Geometry: final body of the model. Coordinates: model frame, mm. A direction names the side the tool comes from. Round coordinates to 2 decimals unless told otherwise and drop trailing zeros. Loops run counter-clockwise (first coordinate to the right, second up) from the corner with the lowest first, then second, coordinate; pieces in that order, holes last. Notation, with made-up numbers: (15, -2) - (26, -2) arc R21 cw to (26, 9) - close; hole circle Ø10 at (16.5, 36). An arc over 180 degrees is marked (long way). Answer in a Markdown table with one row per item. Add a question column.
Autodesk Inventor part; units mm, degrees
ref_plane "YZ Plane" through (0, 0, 0) normal (1, 0, 0) x (0, 1, 0)
ref_plane "XZ Plane" through (0, 0, 0) normal (0, 1, 0) x (-1, 0, 0)
ref_plane "XY Plane" through (0, 0, 0) normal (0, 0, 1) x (1, 0, 0)
sketch "Esboço1" plane through (0, 0, 0) normal (0, 1, 0) x (-1, 0, 0)
  line L0 (50, 50) -> (-50, 50)
  line L1 (-50, 50) -> (-50, -50)
  line L2 (-50, -50) -> (50, -50)
  line L3 (50, -50) -> (50, 50)
  line L4 (-50, 3) -> (-50, -3)
  line L5 (-50, -3) -> (-50, -29)
  line L6 (-50, -29) -> (-50, -50)
  line L7 (-50, -29) -> (-17.5, -29)
  line L8 (-17.5, -29) -> (-17.5, -50)
  line L9 (-50, -50) -> (-50, 50)
  line L10 (-50, 29) -> (-17.5, 29)
  line L11 (-17.5, 29) -> (-17.5, 50)
  line L12 (24.4193, 35) -> (-9.5807, 35)
  line L13 (-9.5807, 35) -> (-9.5807, -35)
  line L14 (-9.5807, -35) -> (24.4193, -35)
  line L15 (24.4193, -35) -> (24.4193, 35)
  line L16 (-33.75, -29) -> (-39.75, -29)
  line L17 (-39.75, -29) -> (-39.75, -3)
  line L18 (-39.75, -3) -> (-33.75, -3)
  line L19 (-33.75, -3) -> (-27.75, -3)
  line L20 (-27.75, -3) -> (-27.75, -29)
  line L21 (-39.75, 29) -> (-39.75, 3)
  line L22 (-39.75, 3) -> (-33.75, 3)
  line L23 (-33.75, 3) -> (-27.75, 3)
  line L24 (-27.75, 3) -> (-27.75, 29)
  line L25 (50, -50) -> (45, -50)
  line L26 (45, -50) -> (45, 50)
  line L27 (45, 0) -> (42, 0)
  line L28 (-17.5, -29) -> (-14.5, -29)
  line L29 (-14.5, -29) -> (-14.5, -47)
  line L30 (-47, 29) -> (-47, -29)
  line L31 (54.9347, -47) -> (45, -47)
  line L32 (24.4193, -47) -> (-14.5, -47)
  line L33 (-17.5, 29) -> (-14.5, 29)
  line L34 (-14.5, 29) -> (-14.5, 47)
  line L35 (-47, -29) -> (-47, 29)
  line L36 (24.4193, 47) -> (-14.5, 47)
  line L37 (-50, 0) -> (-93.4603, 0)
  line L38 (-76.1073, 0) -> (-50, 0)
  line L39 (-47, 0) -> (56.946, 0)
  line L40 (24.4193, 50) -> (24.4193, -47)
  line L41 (93.4603, 0) -> (45, 0)
  line L42 (24.4193, 0) -> (-47, 0)
  line L43 (24.4193, -47) -> (24.4193, -50)
  line L44 (-17.5, 29) -> (-22.5, 29)
  line L45 (-22.5, 29) -> (-22.5, 26)
  line L46 (-22.5, 26) -> (-14.5, 26)
  line L47 (-14.5, 26) -> (-14.5, 29)
  line L48 (-14.5, -29) -> (-14.5, -26)
  line L49 (-17.5, -29) -> (-22.5, -29)
  line L50 (-22.5, -26) -> (-14.5, -26)
  line L51 (-22.5, -26) -> (-22.5, -29)
  point P0 (0, 0)
  point P1 (7.4193, 0)
  point P2 (42, 50)
  point P3 (-9.5807, 0)
  point P4 (42, -50)
  dimension "d0" = 100
  dimension "d1" = 100
  dimension "d2" = 6
  dimension "d3" = 26
  dimension "d4" = 21
  dimension "d5" = 32.5
  dimension "d6" = 34
  dimension "d10" = 26
  dimension "d12" = 10.25
  dimension "d13" = 67.5
  dimension "d14" = 5
  dimension "d17" = 58
  dimension "d18" = 15
  dimension "d23" = 12
  dimension "d24" = 5
  dimension "d25" = 3
  dimension "d26" = 3
extrude "Extrusão1" add sketch "Esboço1" along normal blind 3 contours L26 L27 L39 L15 L40 L0 | L40 L36 L34 L33 L11 L0 | L26 L2 L43 L40 L15 L39 L27 | L40 L12 L13 L39 L30 L10 L21 L22 L23 L24 L45 L46 L47 L34 L36 | L33 L47 L46 L45 L10 | L15 L39 L13 L12 | L15 L14 L13 L39 | L10 L30 L7 L1 | L2 L8 L28 L29 L32 L43 | L40 L32 L29 L48 L50 L51 L7 L20 L19 L18 L17 L30 L39 L13 L14 | L24 L23 L22 L21 L10 | L7 L51 L50 L48 L28 | L17 L18 L19 L20 L7
extrude "Extrusão2" add sketch "Esboço1" against normal blind 35 contours L40 L36 L34 L33 L11 L0 | L33 L47 L46 L45 L10 | L10 L30 L7 L1 | L2 L8 L28 L29 L32 L43 | L7 L51 L50 L48 L28
sketch "Esboço2" plane through (-45, 3, 50) normal (0, 0, 1) x (1, 0, 0)
  line L0 (0, -3) -> (0, 0)
  line L1 (0, -3) -> (13.7317, -11.9575)
  line L2 (0, -3) -> (-4.5989, 0)
  line L3 (-4.5989, 0) -> (0, 0)
  line L4 (20.5807, -3) -> (20.5807, -38)
  line L5 (13.7317, -11.9575) -> (20.5807, -38)
  line L6 (0, 0) -> (0, -3)
  line L7 (0, -3) -> (20.5807, -3)
  line L8 (0, -3) -> (20.5807, -3)
  line L9 (59.5, -3) -> (20.5807, -3)
  line L10 (20.5807, -3) -> (20.5807, -38)
  point P0 (45, -3)
extrude "Extrusão3" add sketch "Esboço2" against normal blind 100
sketch "Esboço5" plane through (17.5, -35, 50) normal (0, 0, 1) x (1, 0, 0)
  line L0 (-41.9193, 0) -> (0, 0)
  line L1 (-41.9193, 0) -> (-4.8193, 0)
  line L2 (32.5, 0) -> (32.5, 38)
  line L3 (-4.8193, 0) -> (32.5, 0)
  line L4 (32.5, 0) -> (32.5, 3)
  line L5 (32.5, 3) -> (-4.8193, 3)
  line L6 (-4.8193, 3) -> (-4.8193, 0)
  point P0 (-17.5, 35)
  dimension "d31" = 37.1
  dimension "d32" = 3
extrude "Extrusão4" cut sketch "Esboço5" against normal blind 100.25
extrude "Extrusão5" add sketch "Esboço5" against normal blind 100
sketch "Esboço6" plane through (50, -35, -50) normal (0, 0, -1) x (-1, 0, 0)
  line L0 (37.3193, 0) -> (74.4193, 0)
  line L1 (74.4193, 0) -> (81.2683, 26.0425)
  line L2 (74.4193, 0) -> (74.4193, -20)
  line L3 (74.4193, 0) -> (0, 0)
  line L4 (0, 0) -> (0, -15)
  line L5 (0, -15) -> (74.4193, -20)
  line L6 (74.4193, 0) -> (0, 0)
  point P0 (50, 35)
  dimension "d37" = 20
  dimension "d38" = 15
extrude "Extrusão6" add sketch "Esboço6" against normal blind 3
mirror "Espelhar1" about plane through (0, 0, 0) normal (0, 0, 1) of "Extrusão6"
sketch "Esboço7" plane through (0, -35, 0) normal (0, -1, 0) x (1, 0, 0)
  line L0 (50, -50) -> (50, -47)
  line L1 (50, -47) -> (47, -47)
  line L2 (-24.4193, -47) -> (50, -47)
  line L3 (47, -47) -> (47, 47)
  line L4 (-24.4193, 47) -> (50, 47)
  line L5 (47, 47) -> (50, 47)
  line L6 (50, 50) -> (50, 29)
  line L7 (50, 47) -> (50, -47)
  point P0 (0, 0)
  dimension "d41" = 3
extrude "Extrusão7" add sketch "Esboço7" along normal blind 15
sketch "Esboço8" plane through (14.5, 0, 47) normal (0, 0, -1) x (-1, 0, 0)
  line L0 (38.9193, -35) -> (38.9193, -55)
  line L1 (38.9193, -35) -> (35.9193, -35)
  line L2 (35.9193, -35) -> (35.9193, -54.7984)
  line L3 (38.9193, -55) -> (-35.5, -50)
  line L4 (35.9193, -54.7984) -> (38.9193, -55)
  line L5 (38.9193, -55) -> (38.9193, -35)
  line L6 (45.7683, -8.9575) -> (64.0989, 3)
  line L7 (38.9193, -35) -> (45.7683, -8.9575)
  line L8 (45.7683, -8.9575) -> (38.9193, -35)
  line L9 (33.7508, -54.6527) -> (44.0879, -15.3473)
  line L10 (33.7508, -54.6527) -> (38.9193, -55)
  line L11 (38.9193, -35) -> (38.9193, -55)
  line L12 (38.9193, 0) -> (38.9193, -35)
  line L13 (38.9193, -55) -> (38.9193, -35)
  point P0 (14.5, 0)
  dimension "d44" = 3
extrude "Extrusão8" cut sketch "Esboço8" along normal mid plane 260.75 contours L0 L3 L2 L9 | L2 L3 L9
sketch "Esboço9" plane through (14.5, 0, 47) normal (0, 0, -1) x (-1, 0, 0)
  line L0 (33.7508, -54.6527) -> (38.9193, -35)
  line L1 (33.7508, -54.6527) -> (30.7576, -54.4516)
  line L2 (33.7508, -54.6527) -> (-35.5, -50)
  line L3 (38.9193, -23.6948) -> (30.7576, -54.4516)
  line L4 (38.9193, -35) -> (38.9193, -23.6948)
  line L5 (38.9193, 0) -> (38.9193, -35)
  line L6 (38.9193, -35) -> (33.7508, -54.6527)
  line L7 (33.7508, -54.6527) -> (30.7576, -54.4516)
  point P0 (14.5, 0)
  dimension "d47" = 3
extrude "Extrusão9" add sketch "Esboço9" along normal blind 95.75
fillet "Arredondamento1" radius 27.75 1 edges at (-31.2683, -8.9575, 0)
properties part number "Peçams2"
1) Section C-C, the plane z = 22.5. Return the cut outline in (x, y).
2) Reachability of faces 4 (the flat face through (17.5, -15, -39)), 5 (the flat face through (22.5, -16, -27)), 6 (the flat face through (17.5, -15, 39)), 7 (the flat face through (19, -16, 26)) from +Z, -Z, +X, -X, +Y, -Y: full face, straight path, thin tool, end or side. Return the list, or none.
3) Section D-D, the plane y = -37. Return the cut outline in (x, z), and give its area (3 significant figures).
4) Pull-direction query (X, two-part tool) for faces 1 (the flat face through (50, -29, 1)), 2 (the flat face through (48, -50, 1)), 3 (the flat face through (12.681, -33, 1)); classes: pulls with the +X half, pulls with the -X half, needs draft (parallel to the pull), parting line crosses it, or undercut.
5) Material intervals for line 1 along Z through (x, y) = (-1, -2); line 2 along Y through (x, z) = (16, 1.5); line 3 along Z through (x, y) = (15, -29), sorted ascending. Write a range as from..to.
6) Section A-A, the plane x = 33.5. Return the cut outline in (y, z), and give its area (3 significant figures).
7) Contact query for flat-ended pins moving along their axis: pin 1 Ø8 at (y, z) = (-46.5, 26) entering from -X; pin 2 Ø10.5 at (y, z) = (-17, -38.5) entering from +X; pin 3 Ø2.5 at (y, z) = (-33, -2.5) entering from -X. Output: stop coordinate, or through.
8) Section B-B, the plane y = -4.5. Return the cut outline in (x, z), and give its area (3 significant figures).
Evaluation:
| question | item | result |
|---|---|---|
| 1 | outline | (-49.6, 3) - (-45, 0) - (-40.22, -3.12) arc R27.75 cw to (-28.55, -19.3) - (-24.42, -35) - (-19.25, -54.65) - (-16.26, -54.45) - (-24.42, -23.69) - (-24.42, 0) - (47, 0) - (47, -32) - (12.68, -32) - (12.68, -35) - (47, -35) - (47, -50) - (50, -50) - (50, 3) - close |
| 2 | face 4 | -Z, +X, +Y |
| 2 | face 5 | +Z, -Z |
| 2 | face 6 | +Z, +X, +Y |
| 2 | face 7 | none |
| 3 | outline | (-23.89, -50) - (50, -50) - (50, 50) - (-23.89, 50) - (-23.89, -47) - close; hole (-20.89, -47) - (47, -47) - (47, 47) - (-20.89, 47) - close |
| 3 | area | 1,010 mm² |
| 4 | face 1 | pulls with the +X half |
| 4 | face 2 | needs draft |
| 4 | face 3 | undercut |
| 5 | line 1 | z = -50..-47, 47..50 |
| 5 | line 2 | y = -35..-32, 0..3 |
| 5 | line 3 | z = -50..-26, 26..50 |
| 6 | outline | (-51.11, -50) - (-32, -50) - (-32, 50) - (-51.11, 50) - (-51.11, 47) - (-35, 47) - (-35, -47) - (-51.11, -47) - close; (0, -29) - (3, -29) - (3, 29) - (0, 29) - close |
| 6 | area | 571 mm² |
| 7 | pin 1 | stops at x = -22.45 |
| 7 | pin 2 | stops at x = 17.5 |
| 7 | pin 3 | stops at x = -25.27 |
| 8 | outline | (-38.29, -50) - (17.5, -50) - (17.5, -29) - (22.5, -29) - (22.5, -26) - (14.5, -26) - (14.5, -47) - (-24.42, -47) - (-24.42, 47) - (14.5, 47) - (14.5, 26) - (22.5, 26) - (22.5, 29) - (17.5, 29) - (17.5, 50) - (-38.29, 50) - close; (47, -29) - (50, -29) - (50, 29) - (47, 29) - close |
| 8 | area | 1,970 mm² |
